```python
from build123d import *

# Parameters (mm, degrees)
SKETCH_1_R          = 25
EXTRUDE_1_DEPTH     = 60
SKETCH_2_R          = 22
CUT_EXTRUDE_1_DEPTH = 55
SKETCH_3_R          = 22
SKETCH_3_R_2        = 15
EXTRUDE_2_DEPTH     = 3


with BuildPart() as part:
    # 草图1 → 凸台-拉伸1 (new body)
    with BuildSketch(Plane(origin=(0, 0, 0), x_dir=(1, 0, 0), z_dir=(0, 1, 0))):
        with Locations(Location((0, 0, 0), (0, 0, 270))):
            Circle(SKETCH_1_R)
    extrude(amount=EXTRUDE_1_DEPTH)

    # 草图2 → 切除-拉伸1 (cut)
    with BuildSketch(Plane.XZ):
        with Locations(Location((0, 0, 0), (0, 0, 270))):
            Circle(SKETCH_2_R)
    extrude(amount=-CUT_EXTRUDE_1_DEPTH, mode=Mode.SUBTRACT)

    # 草图3 → 凸台-拉伸2 (add)
    with BuildSketch(Plane.XZ):
        with Locations(Location((0, 0, 0), (0, 0, 270))):
            Circle(SKETCH_3_R)
        with Locations(Location((0, 0, 0), (0, 0, 270))):
            Circle(SKETCH_3_R_2, mode=Mode.SUBTRACT)
    extrude(amount=-EXTRUDE_2_DEPTH)


solid = part.part
```
CAD build for the part. Positions are in the model's coordinates, mm. A direction names the side the tool comes from. Coordinates: 2 decimals unless noted, no trailing zeros. Order: outer loops, then holes, each group sorted by start corner. A loop starts at its lowest first (then second) coordinate and runs counter-clockwise, first axis right, second up.
(1) Pin check, flat tips, straight feed: pin 1 Ø2 at (x, y) = (-12, 39) entering from -Z; pin 2 Ø4 at (x, y) = (-6.5, 17.5) entering from -Z; pin 3 Ø1.5 at (y, z) = (42.5, -18.5) entering from -X; pin 4 Ø1 at (x, y) = (-0.5, 27.5) entering from -Z. Stop position of each tip, or through.
Solution:
pin 1: stops at z = -22.45
pin 2: stops at z = -24.59
pin 3: stops at x = -17.61
pin 4: stops at z = -25
(2) Drill centre lines: L1, parallel to Y at x = -16, z = -3.5; L2, parallel to X at y = 22.5, z = 0; L3, parallel to X at y = 2.05, z = 0. Where is each one in solid material? Low to high.
Solution:
L1: y = 0 to 3, 55 to 60
L2: x = -25 to -22, 22 to 25
L3: x = -25 to -15, 15 to 25
(3) Saw through at C-C, the plane y = 49. Write the cut outline in (x, z), and give its area (3 significant figures).
Solution:
outline: circle Ø50 at (0, 0); hole circle Ø44 at (0, 0)
area: 443 mm2
(4) Saw through at A-A, the plane x = 0. Write the cut outline in (y, z), and give its area (3 significant figures).
Solution:
outline: (0, -25) - (60, -25) - (60, 25) - (0, 25) - (0, 15) - (3, 15) - (3, 22) - (55, 22) - (55, -22) - (3, -22) - (3, -15) - (0, -15) - close
area: 622 mm2
(5) Mould opens along Z. For faces 3 (the face through (5.2, 3, -14.4)), 4 (the face through (0.66, 1.479, 14.985)), 5 (the face through (0, 60, 0)), 6 (the face through (7.509, 29.58, 23.846)) say: released by +Z, released by -Z, zero draft, split by the parting line, or undercut.
Solution:
face 3: undercut
face 4: undercut
face 5: zero draft
face 6: split by the parting line
(6) Saw through at D-D, the plane x = -21. Write the cut outline in (y, z).
Solution:
outline: (0, -13.56) - (60, -13.56) - (60, 13.56) - (0, 13.56) - close; hole (3, -6.56) - (55, -6.56) - (55, 6.56) - (3, 6.56) - close
(7) Saw through at B-B, the plane z = 18.5. Write the cut outline in (x, y), and give its area (3 significant figures).
Solution:
outline: (-16.82, 0) - (16.82, 0) - (16.82, 60) - (-16.82, 60) - close; hole (-11.91, 3) - (11.91, 3) - (11.91, 55) - (-11.91, 55) - close
area: 780 mm2
(8) Which spindle directions (+Z, -Z, +X, -X, +Y, -Y) get a long thin tool onto all of the face, cutting with end or side? Do faces 1 (the face through (0, 55, 0)), 2 (the face through (-11, 0, -11)). Say none if no direction does.
Solution:
face 1: none
face 2: +Z, -Z, +X, -X, -Y
